The listing builds one solid part. Answer for the finished solid, in the listing's coordinates (mm). Coordinates: 2 decimals unless noted, no trailing zeros. Loops run counter-clockwise (first coordinate to the right, second up) from the corner with the lowest first, then second, coordinate; pieces in that order, holes last. Notation, with made-up numbers: M 86,-39 L 118,-39 A32 ccw 118,-8 Z; hole C 63,-13 d7. An arc over 180 degrees is marked long. Return JSON: item names as keys, results as strings. Group by question number.
1. Section A-A (y = 126) is taken. Write down the section's boundary in (x, z).
2. Given P1, Ø2.5, axis at x = 55, y = 40, coming from the -Z side, flat-ended and moving along its own axis, determine where the tip first touches the part or whether it passes through.
3. The mould has two halves that part along Z. Classify faces 1 (the face through (222, 97, 0)), 2 (the face through (222, 97, 6)): pulls with the +Z half, pulls with the -Z half, needs draft (parallel to the pull), parting line crosses it, or undercut.
4. Section C-C (x = 254.5) is taken. Write down the section's boundary in (y, z), then the cut area to 3 significant figures.
5. Straight lines are drawn through the part: L1, parallel to Y at x = 219, z = 2.7; L2, parallel to X at y = 234, z = 2.9; L3, parallel to X at y = 39.5, z = 4.15. For each, find the intervals that lie inside material, in ascending order. Write a range as from..to.
6. Section B-B (z = 4) is taken. Count the separate pieces of the cut face and the enclosed holes in it, then the cut area to 3 significant figures.
```python
from build123d import *

# Parameters (mm, degrees)
SKETCH_1_R      = 1.5
SKETCH_1_R_2    = 2
EXTRUDE_1_DEPTH = 6


with BuildPart() as part:
    # Эскиз1 → Бобышка-Вытянуть1 (new body)
    with BuildSketch(Plane.XY):
        with BuildLine():
            Line((129, 244), (129, 121.5))
            ThreePointArc((129, 121.5), (131.196699141, 116.196699141), (136.5, 114))
            Line((136.5, 114), (301.5, 114))
            ThreePointArc((301.5, 114), (306.803300859, 116.196699141), (309, 121.5))
            Line((309, 121.5), (309, 244))
            Line((309, 244), (438, 244))
            Line((438, 244), (438, 0))
            Line((438, 0), (0, 0))
            Line((0, 0), (0, 244))
            Line((0, 244), (129, 244))
        make_face()
        with Locations((10, 10)):
            Circle(SKETCH_1_R, mode=Mode.SUBTRACT)
        with Locations((10, 234)):
            Circle(SKETCH_1_R, mode=Mode.SUBTRACT)
        with Locations((121.5, 234)):
            Circle(SKETCH_1_R, mode=Mode.SUBTRACT)
        with Locations((316.5, 234)):
            Circle(SKETCH_1_R, mode=Mode.SUBTRACT)
        with Locations((428, 234)):
            Circle(SKETCH_1_R, mode=Mode.SUBTRACT)
        with Locations((428, 10)):
            Circle(SKETCH_1_R, mode=Mode.SUBTRACT)
        with Locations((219, 106.5)):
            Circle(SKETCH_1_R, mode=Mode.SUBTRACT)
        with Locations((219, 10)):
            Circle(SKETCH_1_R, mode=Mode.SUBTRACT)
        with Locations((333, 70)):
            Circle(SKETCH_1_R_2, mode=Mode.SUBTRACT)
        with Locations((383, 70)):
            Circle(SKETCH_1_R_2, mode=Mode.SUBTRACT)
        with Locations((383, 40)):
            Circle(SKETCH_1_R_2, mode=Mode.SUBTRACT)
        with Locations((333, 40)):
            Circle(SKETCH_1_R_2, mode=Mode.SUBTRACT)
        with Locations((55, 70)):
            Circle(SKETCH_1_R_2, mode=Mode.SUBTRACT)
        with Locations((105, 70)):
            Circle(SKETCH_1_R_2, mode=Mode.SUBTRACT)
        with Locations((55, 40)):
            Circle(SKETCH_1_R_2, mode=Mode.SUBTRACT)
        with Locations((105, 40)):
            Circle(SKETCH_1_R_2, mode=Mode.SUBTRACT)
    extrude(amount=EXTRUDE_1_DEPTH)


solid = part.part
```
Worked out:
{
 "1": {"outline": "M 0,0 L 129,0 L 129,6 L 0,6 Z; M 309,0 L 438,0 L 438,6 L 309,6 Z"},
 "2": {"P1": "through"},
 "3": {"face 1": "pulls with the -Z half", "face 2": "pulls with the +Z half"},
 "4": {"outline": "M 0,0 L 114,0 L 114,6 L 0,6 Z", "area": "684 mm^2"},
 "5": {"L1": "0..8.5, 11.5..105, 108..114", "L2": "0..8.5, 11.5..120, 123..129, 309..315, 318..426.5, 429.5..438", "L3": "0..53.06, 56.94..103.06, 106.94..331.06, 334.94..381.06, 384.94..438"},
 "6": {"separate pieces": "1", "enclosed holes": "16", "area": "83,300 mm^2"}
}
